Autodesk Inventor part; units mm, degrees
ref_plane "Work Plane3" through (6.309, 11.7147, -0.85) normal (-0.866, -0.5, 0) x (0.5, -0.866, 0)
ref_plane "XY Plane" through (0, 0, 0) normal (0, 0, 1) x (1, 0, 0)
sketch "Sketch1" plane through (0, 0, 0) normal (0, 1, 0) x (-1, 0, 0)
  line L0 (0, -0.13) -> (17.417, -0.13)
  line L1 (17.417, -0.13) -> (17.417, 0.13)
  line L2 (17.417, 0.13) -> (0, 0.13)
  line L3 (0, 0.13) -> (0, -0.13)
  line L4 (-17.289, 0) -> (34.651, 0) construction
  line L5 (22.681, -3.5) -> (-5.169, -3.5)
  line L6 (-5.169, -3.5) -> (-5.169, 4)
  line L7 (-5.169, 4) -> (22.681, 4)
  line L8 (22.681, 4) -> (22.681, -3.5)
  line L9 (27.231, -2.85) -> (-9.869, -2.85) construction
  line L10 (-9.869, -2.85) -> (-9.869, -0.85) construction
  line L11 (-9.869, -0.85) -> (27.231, -0.85) construction
  line L12 (27.231, -0.85) -> (27.231, -2.85) construction
  point P0 (0, 0)
  dimension "d1" = 17.417
  dimension "d2" = 0.26
  dimension "d7" = 7.5
  dimension "d8" = 27.85
  dimension "d9" = 0.85
  dimension "d10" = 2
  dimension "d11" = 9.814
  dimension "d12" = 37.1
  dimension "d13" = 4.55
  dimension "d20" = 4.85
ref_plane "Alu_Start_V" through (0, 2.27, 0) normal (0, 1, 0) x (-1, 0, 0)
sketch "Sketch2" plane through (0, 2.27, 0) normal (0, 1, 0) x (-1, 0, 0)
  line L0 (27.231, -2.85) -> (-9.869, -2.85)
  line L1 (27.231, -0.85) -> (27.231, -2.85)
  line L2 (-9.869, -0.85) -> (27.231, -0.85)
  line L3 (-9.869, -2.85) -> (-9.869, -0.85)
  point P0 (0, 0)
extrude "Extrusion2" add sketch "Sketch2" along normal blind 38
extrude "Extrusion3" add sketch "Sketch1" along normal blind 1.64 contours L3 L2 L1 L0 | L5 L6 L7 L8
sketch "Sketch3" plane through (0, 1.64, 0) normal (0, 1, 0) x (1, 0, 0)
  line L0 (5.169, 4.5) -> (-22.681, 4.5)
  line L1 (-22.681, 4.5) -> (-22.681, 0.85)
  line L2 (-22.681, 0.85) -> (5.169, 0.85)
  line L3 (5.169, 0.85) -> (5.169, 4.5)
  line L4 (9.869, 2.85) -> (-27.231, 2.85) construction
  line L5 (-27.231, 0.85) -> (9.869, 0.85) construction
  point P0 (0, 0)
  point P1 (-22.681, 3.5)
  point P2 (5.169, 3.5)
  point P3 (-22.681, 2.85)
  point P4 (5.169, 2.85)
  dimension "d22" = 3.65
extrude "Extrusion4" add sketch "Sketch3" along normal up to surface (0.63 mm away)
sketch "NozzleLine" plane through (0, 0, 0) normal (0, -1, 0) x (1, 0, 0)
  line L0 (0, 0) -> (-17.417, 0)
  point P0 (-17.417, 0.13)
  point P1 (-8.7085, 0)
sketch "Sketch5" plane through (9.869, 40.27, -2.85) normal (0, 0, -1) x (-1, 0, 0)
  line L0 (0, -38) -> (0, 0)
  line L1 (0, -10.64) -> (1.35, -10.64)
  arc A0 (1.35, -13.34) -> (1.35, -10.64) centre (1.35, -11.99) ccw
  line L2 (1.35, -13.34) -> (0, -13.34)
  line L3 (37.1, 0) -> (0, 0) construction
  line L4 (4.7, -38) -> (32.55, -38) construction
  line L5 (37.1, -38) -> (37.1, 0) construction
  line L6 (18.55, 0) -> (18.55, -38) construction
  line L7 (37.1, -10.64) -> (35.75, -10.64)
  arc A1 (35.75, -10.64) -> (35.75, -13.34) centre (35.75, -11.99) ccw
  line L8 (35.75, -13.34) -> (37.1, -13.34)
  line L9 (0, -22.99) -> (36.8238, -22.99) construction
  line L10 (0, -35.34) -> (1.35, -35.34)
  arc A2 (1.35, -35.34) -> (1.35, -32.64) centre (1.35, -33.99) ccw
  line L11 (1.35, -32.64) -> (0, -32.64)
  line L12 (37.1, -45.98) -> (0, -45.98) construction
  line L13 (37.1, -35.34) -> (35.75, -35.34)
  arc A3 (35.75, -32.64) -> (35.75, -35.34) centre (35.75, -33.99) ccw
  line L14 (35.75, -32.64) -> (37.1, -32.64)
  line L15 (37.1, -10.64) -> (37.1, -13.34)
  line L16 (37.1, -32.64) -> (37.1, -35.34)
  line L17 (-7.42, -38) -> (44.52, -38)
  point P0 (9.869, -40.27)
  point P1 (18.55, -45.98)
  point P2 (0, -32.64)
  point P3 (0, -35.34)
  dimension "d25" = 2.7
  dimension "d28" = 2.7
  dimension "d38" = 4.01
  dimension "d39" = 26.01
extrude "Extrusion5" cut sketch "Sketch5" against normal through all
ref_plane "NozzleLineCenter" through (-8.7085, 0, 0) normal (1, 0, 0) x (0, 1, 0)
sketch "Sketch6" plane through (-27.231, 40.27, -0.85) normal (0, 0, 1) x (1, 0, 0)
  line L0 (33.54, -28.5553) -> (35.09, -31.24)
  line L1 (4.55, -40.27) -> (32.4, -40.27)
  line L2 (37.1, -38) -> (37.1, -35.34)
  line L3 (32.4, -40.27) -> (4.55, -40.27)
  line L4 (37.1, -32.64) -> (37.1, -13.34)
  line L5 (-7.42, -38) -> (44.52, -38)
  line L6 (35.09, -31.24) -> (30.5153, -33.8812)
  point P0 (27.231, -40.27)
  dimension "d33" = 3.1
  dimension "d37" = 2.01
  dimension "d40" = 6.76
  dimension "d41" = 30
ref_plane "Work Plane3" through (6.309, 11.7147, -0.85) normal (-0.866, -0.5, 0) x (0.5, -0.866, 0)
sketch "Sketch7" plane through (6.309, 11.7147, -0.85) normal (-0.866, -0.5, 0) x (0.5, -0.866, 0)
  circle A0 centre (1.55, 5.2) radius 1.55
  line L0 (0, 0) -> (3.1, 0) construction
  line L1 (1.55, 5.2) -> (1.55, 0) construction
  point P0 (6.9907, 0.85)
  dimension "d43" = 3.1
  dimension "d45" = 5.2
extrude "Extrusion6" add sketch "Sketch7" along normal up to surface surface through (-8.756, 1.64, 0.25) normal (0, 1, 0)
properties part number "Xaar128"
The listing builds one solid part. Answer for the finished solid, in the listing's coordinates (mm). A direction names the side the tool comes from. Round coordinates to 2 decimals unless told otherwise and drop trailing zeros. Write each loop counter-clockwise with the first axis right and the second up, starting at its lowest first coordinate (ties: lowest second). Pieces come first, ordered by that corner, then holes. Notation, with made-up numbers: M -39,-35.5 L -27,-35.5 A14 ccw -27,-31.5 Z; hole C 30,87 d4. An arc over 180 degrees is marked long. Write each question's results on one line, items separated by ' | '. Start each with the question number.
Item 1: Find section B-B on y = 28.28. Write down the section's boundary in (x, z).
Item 2: The mould has two halves that part along Y. Classify faces 5 (the flat face through (-25, 2.27, -2)), 6 (the flat face through (9, 4.93, -2)), 7 (the flat face through (7.073, 10.391, 4.372)): +Y half, -Y half, draft (parallel to the pull), parting line (faces both ways), or undercut.
Item 3: Straight lines are drawn through the part: probe 1 along Y at (x, z) = (-21, -0.5); probe 2 along Z at (x, y) = (7.5, 26.5); probe 3 along Y at (x, z) = (7.5, -2). For each, find the intervals that lie inside material, in ascending order.
Item 4: Given pin 1 Ø1 at (x, z) = (-24.5, -1.5) entering from -Y; pin 2 Ø2 at (x, y) = (5.5, 7) entering from -Z; pin 3 Ø1.1 at (x, z) = (-9, -4) entering from -Y; pin 4 Ø11 at (x, y) = (-5.5, 15) entering from +Z, each flat-ended and moving along its own axis, determine where each tip first touches the part or whether it passes through.
Item 5: Find section C-C on z = 5.25. Write down the section's boundary in (x, y), and give its area (3 significant figures).
Item 6: Find section A-A on x = -18. Write down the section's boundary in (y, z).
Item 7: Which of the six approach directions +Z, -Z, +X, -X, +Y, -Y give full straight-line access (tool end or side, diameter ignored) to faces 1 (the flat face through (8, 2.27, -2)), 2 (the flat face through (9, 7.63, -2)), 3 (the flat face through (-27, 4.93, -2)), 4 (the flat face through (-9, 21, -2.85))?
Answer block:
1) outline: M -24.53,-2.85 L 7.17,-2.85 L 7.17,-0.85 L -24.53,-0.85 Z
2) face 5: -Y half | face 6: undercut | face 7: +Y half
3) probe 1: y = 0 to 1.64 | probe 2: z = -2.85 to -0.85 | probe 3: y = 2.27 to 5.39, 7.17 to 27.39, 29.17 to 40.27
4) pin 1: stops at y = 2.27 | pin 2: stops at z = -2.85 | pin 3: stops at y = 0 | pin 4: stops at z = -0.85
5) outline: M -10.56,1.64 L -5.52,1.64 L 7.71,9.28 L 6.45,11.47 Z | area: 44.1 mm²
6) outline: M 0,-3.5 L 1.64,-3.5 L 1.64,-4.5 L 2.27,-4.5 L 2.27,-2.85 L 40.27,-2.85 L 40.27,-0.85 L 1.64,-0.85 L 1.64,4 L 0,4 Z
7) face 1: +Z, -Z, +X, -Y | face 2: +Z, -Z, +X | face 3: +Z, -Z, -X | face 4: -Z, +X, -X, +Y
